from build123d import *

# Parameters (mm, degrees)
SKETCH_1_W          = 15
SKETCH_1_H          = 60
EXTRUDE_1_DEPTH     = 55
CUT_EXTRUDE_1_DEPTH = 53
SKETCH_3_W          = 78.566437997
SKETCH_3_H          = 30
CUT_EXTRUDE_2_DEPTH = 35
CUT_EXTRUDE_3_DEPTH = 25
FILLET_1_R          = 2
SKETCH_5_R          = 1.75
CUT_EXTRUDE_4_DEPTH = 3
SKETCH_6_R          = 1.75
CUT_EXTRUDE_5_DEPTH = 3
SKETCH_7_R          = 1.75
CUT_EXTRUDE_6_DEPTH = 3
SKETCH_8_W          = 60
SKETCH_8_H          = 7
CUT_EXTRUDE_7_DEPTH = 68.625993731
SKETCH_9_R          = 1.75
CUT_EXTRUDE_8_DEPTH = 10
SKETCH_10_W         = 8.867546431
SKETCH_10_H         = 10.62822389
CUT_EXTRUDE_9_DEPTH = 78


with BuildPart() as part:
    # 草图1 → 凸台-拉伸1 (new body)
    with BuildSketch(Plane(origin=(0, 0, 0), x_dir=(1, 0, 0), z_dir=(0, 1, 0))):
        Polygon((-7.5, 30), (-32.672988935, 0), (-7.5, -30), align=None)
        Rectangle(SKETCH_1_W, SKETCH_1_H)
    extrude(amount=EXTRUDE_1_DEPTH)

    # 草图2 → 切除-拉伸1 (cut)
    with BuildSketch(Plane(origin=(0, 55, 0), x_dir=(1, 0, 0), z_dir=(0, 1, 0))):
        Polygon((-6.334230855, 27.5), (-29.409470712, 0), (-6.334230855, -27.5), (5, -27.5), (5, 27.5), align=None)
    extrude(amount=-CUT_EXTRUDE_1_DEPTH, mode=Mode.SUBTRACT)

    # 草图3 → 切除-拉伸2 (cut)
    with BuildSketch(Plane(origin=(0, 55, 0), x_dir=(1, 0, 0), z_dir=(0, 1, 0))):
        with Locations((-12.586494467, 0)):
            Rectangle(SKETCH_3_W, SKETCH_3_H)
    extrude(amount=-CUT_EXTRUDE_2_DEPTH, mode=Mode.SUBTRACT)

    # 草图4 → 切除-拉伸3 (cut)
    with BuildSketch(Plane(origin=(0, 20, 0), x_dir=(1, 0, 0), z_dir=(0, 1, 0))):
        Polygon((-16.822976244, 15), (-73.584466249, 15), (-53.824577323, -15), (-16.822976244, -15), align=None)
    extrude(amount=-CUT_EXTRUDE_3_DEPTH, mode=Mode.SUBTRACT)

    # 圆角1
    # the kernel refuses this fillet: 2 mm, written as the material it takes off along each edge
    with BuildSketch(Plane(origin=(-20.086494468, 65.085601878, 15), x_dir=(1, 0, 0), z_dir=(0, -1, 0))) as fillet_1_piece_1:
        with BuildLine():
            CenterArc((4.125248856, 1.80483249), FILLET_1_R, 140, 104.477512186)
            Line((2.593159969, 3.09040771), (2.562518192, 3.116119214))
            Line((2.562518192, 3.116119214), (-0.030641778, 0.025711504))
            Line((-0.030641778, 0.025711504), (0, -0.04))
            ThreePointArc((0, -0.04), (1.631759112, -0.04), (3.246283611, -0.03609665))
            Line((3.246283611, -0.03609665), (3.263518223, 0))
        make_face()
    extrude(amount=75.171203755, mode=Mode.SUBTRACT)
    with BuildSketch(Plane(origin=(-20.086494468, -10.085601878, -15), x_dir=(0.6427876096865405, 0, -0.7660444431189769), z_dir=(0, 1, 0))) as fillet_1_piece_2:
        with BuildLine():
            CenterArc((4.034240751, -2), FILLET_1_R, 90, 104.477512186)
            Line((2.097749078, -2.5), (2.059019244, -2.51))
            ThreePointArc((2.059019244, -2.51), (1.018232761, -1.275711504), (-0.030641778, -0.025711504))
            Line((-0.030641778, -0.025711504), (0, 0.04))
            Line((0, 0.04), (4.034240751, 0.04))
            Line((4.034240751, 0.04), (4.034240751, 0))
        make_face()
    extrude(amount=75.171203755, mode=Mode.SUBTRACT)

    # 草图5 → 切除-拉伸4 (cut)
    with BuildSketch(Plane(origin=(-19.173296961, 0, 16.088306409), x_dir=(0.6427876096865413, 0, 0.7660444431189765), z_dir=(-0.7660444431189765, 0, 0.6427876096865413))):
        with Locations((7.613557632, 44)):
            Circle(SKETCH_5_R)
        with Locations((6.613557632, 6.513335705)):
            Circle(SKETCH_5_R)
    extrude(amount=-CUT_EXTRUDE_4_DEPTH, mode=Mode.SUBTRACT)

    # 草图6 → 切除-拉伸5 (cut)
    with BuildSketch(Plane(origin=(-19.173296961, 0, -16.088306409), x_dir=(-0.642787609686541, 0, 0.7660444431189768), z_dir=(-0.7660444431189768, 0, -0.642787609686541))):
        with Locations((-7.613557632, 44)):
            Circle(SKETCH_6_R)
        with Locations((-7.613557632, 6.5)):
            Circle(SKETCH_6_R)
    extrude(amount=-CUT_EXTRUDE_5_DEPTH, mode=Mode.SUBTRACT)

    # 草图7 → 切除-拉伸6 (cut)
    with BuildSketch(Plane(origin=(7.5, 0, 0), x_dir=(0, 0, -1), z_dir=(1, 0, 0))):
        with Locations((18.75, 10)):
            Circle(SKETCH_7_R)
        with Locations(Location((-18.75, 10, 0), (0, 0, 180))):
            Circle(SKETCH_7_R)
    extrude(amount=-CUT_EXTRUDE_6_DEPTH, mode=Mode.SUBTRACT)

    # 草图8 → 切除-拉伸7 (cut, through all)
    with BuildSketch(Plane(origin=(7.5, 0, 0), x_dir=(0, 0, -1), z_dir=(1, 0, 0))):
        with Locations((0, 51.5)):
            Rectangle(SKETCH_8_W, SKETCH_8_H)
    extrude(amount=-CUT_EXTRUDE_7_DEPTH, mode=Mode.SUBTRACT)

    # 草图9 → 切除-拉伸8 (cut)
    with BuildSketch(Plane(origin=(0, 2, 0), x_dir=(1, 0, 0), z_dir=(0, 1, 0))):
        with Locations(Location((-0.667115427, -23.5, 0), (0, 0, 270))):
            Circle(SKETCH_9_R)
        with Locations(Location((-0.667115427, 23.5, 0), (0, 0, 270))):
            Circle(SKETCH_9_R)
    extrude(amount=-CUT_EXTRUDE_8_DEPTH, mode=Mode.SUBTRACT)

    # 草图10 → 切除-拉伸9 (cut)
    with BuildSketch(Plane.XY.offset(30)):
        with Locations((3.066226785, 42.685888055)):
            Rectangle(SKETCH_10_W, SKETCH_10_H)
    extrude(amount=-CUT_EXTRUDE_9_DEPTH, mode=Mode.SUBTRACT)


solid = part.part
Design review of the part built by this model. Coordinates are the model's own, in mm. A direction names the side the tool comes from. Coordinates: 2 decimals unless noted, no trailing zeros. Write each loop counter-clockwise with the first axis right and the second up, starting at its lowest first coordinate (ties: lowest second). Pieces come first, ordered by that corner, then holes. Notation, with made-up numbers: (-30, -5.75) -> (-19, -5.75) arc R12 ccw to (-19, 5.25) -> close; hole circle Ø4 at (54, -28.5). An arc over 180 degrees is marked (long way). Write each question's results on one line, items separated by ' | '. Start each with the question number.
(1) For line 1 along Y through (x, z) = (6.45, -18.75); line 2 along Z through (x, y) = (-3.25, 17.5); line 3 along Y through (x, z) = (2.5, -15), list the stretches that pass through material, from the lowest coordinate up. Write a range as from..to.
(2) The part is to be moulded in two halves that separate along Z. For faces 1 (the face through (6, 29, 15)), 2 (the face through (0, 24, 30)), 3 (the face through (-10, 48, -24)), 4 (the face through (-11.505, 25.322, -21.337)), say which applies: pulls with the +Z half, pulls with the -Z half, needs draft (parallel to the pull), parting line crosses it, or undercut.
(3) Take a section at C-C on z = 0. Write out the cut boundary in (x, y), and give its area (3 significant figures).
(4) Tool access review of faces 5 (the face through (6, 37.372, 26)), 6 (the face through (-6, 2, 0)), 7 (the face through (6.27, 11.18, -17.46)): name each direction out of +Z, -Z, +X, -X, +Y, -Y from which nothing blocks a thin tool from reaching the whole face with its end or side.
(5) Take a section at B-B on y = 10. Write out the cut boundary in (x, z).
(6) Clearance check with flat-ended pins moving along their axes: P1, Ø10, axis at x = 1, z = 1, coming from the +Y side; P2, Ø7, axis at x = 4.5, z = -22.5, coming from the +Y side; P3, Ø1.5, axis at x = -12.5, y = 36.5, coming from the -Z side. State where each tip first meets the part, or that it passes through.
(7) Take a section at A-A on y = 38.5. Write out the cut boundary in (x, z), and give its area (3 significant figures).
(8) Take a section at D-D on y = 17. Write out the cut boundary in (x, z), and give its area (3 significant figures).
Results found:
1) line 1: y = 0..8.25, 11.75..37.37 | line 2: z = -30..-27.5, 27.5..30 | line 3: y = 0..2
2) face 1: undercut | face 2: pulls with the +Z half | face 3: needs draft | face 4: undercut
3) outline: (-16.82, 0) -> (7.5, 0) -> (7.5, 20) -> (5, 20) -> (5, 2) -> (-16.82, 2) -> close | area: 93.6 mm2
4) face 5: +Z, -Z, +X, +Y | face 6: +Y | face 7: +X
5) outline: (-17.49, -18.09) -> (-7.5, -30) -> (7.5, -30) -> (7.5, -20.5) -> (5, -20.5) -> (5, -27.5) -> (-6.33, -27.5) -> (-16.82, -15) arc R2 ccw to start; (-17.49, 18.09) arc R2 ccw to (-16.82, 15) -> (-6.33, 27.5) -> (5, 27.5) -> (5, 20.5) -> (7.5, 20.5) -> (7.5, 30) -> (-7.5, 30) -> close; (5, -17) -> (7.5, -17) -> (7.5, 17) -> (5, 17) -> close
6) P1: stops at y = 20 | P2: stops at y = 37.37 | P3: stops at z = -24.94
7) outline: (-17.49, -18.09) -> (-7.5, -30) -> (-1.37, -30) -> (-1.37, -27.5) -> (-6.33, -27.5) -> (-16.82, -15) arc R2 ccw to start; (-17.49, 18.09) arc R2 ccw to (-16.82, 15) -> (-6.33, 27.5) -> (-1.37, 27.5) -> (-1.37, 30) -> (-7.5, 30) -> close | area: 111 mm2
8) outline: (-17.49, -18.09) -> (-7.5, -30) -> (7.5, -30) -> (7.5, 30) -> (-7.5, 30) -> (-17.49, 18.09) arc R2 ccw to (-16.82, 15) -> (-6.33, 27.5) -> (5, 27.5) -> (5, -27.5) -> (-6.33, -27.5) -> (-16.82, -15) arc R2 ccw to start | area: 293 mm2
